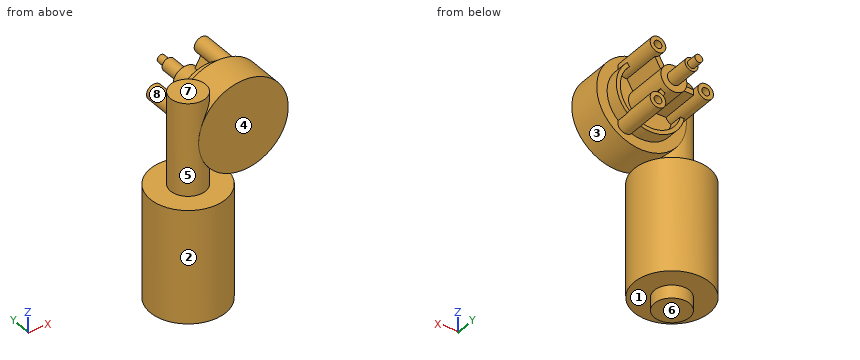
```python
from build123d import *

# Parameters (mm, degrees)
SKETCH1_R           = 29
BOSS_EXTRUDE1_DEPTH = 87
SKETCH3_W           = 13.5
SKETCH3_H           = 168
SKETCH4_R           = 34.5
BOSS_EXTRUDE2_DEPTH = 13.5
SKETCH5_R           = 6
SKETCH5_R_2         = 10
BOSS_EXTRUDE3_DEPTH = 35
BOSS_EXTRUDE4_DEPTH = 30
SKETCH7_R           = 26.5
SKETCH7_R_2         = 23.5
BOSS_EXTRUDE5_DEPTH = 10
SKETCH8_R           = 3
CUT_EXTRUDE1_DEPTH  = 18
SKETCH9_R           = 5
BOSS_EXTRUDE6_DEPTH = 19
SKETCH10_R          = 3
BOSS_EXTRUDE7_DEPTH = 8


with BuildPart() as part:
    # Sketch1 → Boss-Extrude1 (new body)
    with BuildSketch(Plane.XY):
        Circle(SKETCH1_R)
    extrude(amount=BOSS_EXTRUDE1_DEPTH)

    # Sketch3 → Revolve1 (revolve)
    with BuildSketch(Plane(origin=(0, 0, 0), x_dir=(1, 0, 0), z_dir=(0, 1, 0))):
        with Locations((-6.75, -74)):
            Rectangle(SKETCH3_W, SKETCH3_H)
    revolve(axis=Axis((0, 0, 0), (0, 0, 1)))

    # Sketch4 → Boss-Extrude2 (add, symmetric)
    with BuildSketch(Plane(origin=(0, 0, 0), x_dir=(1, 0, 0), z_dir=(0, 1, 0))):
        with Locations((33, -126.5)):
            Circle(SKETCH4_R)
    extrude(amount=BOSS_EXTRUDE2_DEPTH, both=True)

    # Sketch5 → Boss-Extrude3 (add)
    with BuildSketch(Plane(origin=(0, 13.5, 0), x_dir=(1, 0, 0), z_dir=(0, 1, 0))):
        with Locations((8.5, -126.5)):
            Circle(SKETCH5_R)
        with Locations((33, -126.5)):
            Circle(SKETCH5_R_2)
        with Locations((45.25, -105.282377607)):
            Circle(SKETCH5_R)
        with Locations((45.25, -147.717622393)):
            Circle(SKETCH5_R)
    extrude(amount=BOSS_EXTRUDE3_DEPTH)

    # Sketch6 → Boss-Extrude4 (add)
    with BuildSketch(Plane(origin=(0, 13.5, 0), x_dir=(1, 0, 0), z_dir=(0, 1, 0))):
        Polygon((31.845299462, -128.5), (2.843145751, -128.5), (2.843145751, -124.5), (31.845299462, -124.5), (46.346376317, -99.383398122), (49.810477932, -101.383398122), (36.0121545, -125.282795366), (36.116305102, -127.897598768), (49.810477932, -151.616601878), (46.346376317, -153.616601878), align=None)
    extrude(amount=BOSS_EXTRUDE4_DEPTH)

    # Sketch7 → Boss-Extrude5 (add)
    with BuildSketch(Plane(origin=(0, 13.5, 0), x_dir=(1, 0, 0), z_dir=(0, 1, 0))):
        with Locations((33, -126.5)):
            Circle(SKETCH7_R)
        with Locations((33, -126.5)):
            Circle(SKETCH7_R_2, mode=Mode.SUBTRACT)
    extrude(amount=BOSS_EXTRUDE5_DEPTH)

    # Sketch8 → Cut-Extrude1 (cut)
    with BuildSketch(Plane(origin=(0, 48.5, 0), x_dir=(1, 0, 0), z_dir=(0, 1, 0))):
        with Locations((8.5, -126.5)):
            Circle(SKETCH8_R)
        with Locations((45.25, -105.282377607)):
            Circle(SKETCH8_R)
        with Locations((45.25, -147.717622393)):
            Circle(SKETCH8_R)
    extrude(amount=-CUT_EXTRUDE1_DEPTH, mode=Mode.SUBTRACT)

    # Sketch9 → Boss-Extrude6 (add)
    with BuildSketch(Plane(origin=(0, 48.5, 0), x_dir=(1, 0, 0), z_dir=(0, 1, 0))):
        with Locations((33, -126.5)):
            Circle(SKETCH9_R)
    extrude(amount=BOSS_EXTRUDE6_DEPTH)

    # Sketch10 → Boss-Extrude7 (add)
    with BuildSketch(Plane(origin=(0, 67.5, 0), x_dir=(1, 0, 0), z_dir=(0, 1, 0))):
        with Locations((33, -126.5)):
            Circle(SKETCH10_R)
    extrude(amount=BOSS_EXTRUDE7_DEPTH)


solid = part.part
```
Input: part model. Units: mm. Frame: model coordinates. Face numbers are marked on the shaded views. A direction names the side the tool comes from. Coordinates: 2 decimals unless noted, no trailing zeros. Write each loop counter-clockwise with the first axis right and the second up, starting at its lowest first coordinate (ties: lowest second). Pieces come first, ordered by that corner, then holes.
1) Pin query (flat end, axial travel): pin 1 Ø5 at (x, z) = (-13.5, 31.5) entering from +Y; pin 2 Ø6.5 at (x, z) = (44, 106) entering from +Y; pin 3 Ø5 at (x, z) = (54.5, 134.5) entering from +Y. Return the tip coordinate at first contact, or that it passes through.
2) Section C-C on y = -5.5. Output: boundary loops of the cut face in (x, z), and give its area (3 significant figures).
3) Material intervals for line 1 along X through (y, z) = (44, 126); line 2 along Z through (x, y) = (45.25, 37); line 3 along X through (y, z) = (42.5, 126.5), sorted ascending.
4) Set-up query: the marked faces 4, 5, 6, 7 and 8. Return all of +Z, -Z, +X, -X, +Y, -Y with unobstructed straight access to the full face (end or side cutting, diameter ignored); none if empty.
5) Section D-D on z = 2. Output: boundary loops of the cut face in (x, y).
6) Section B-B on y = 18.5. Output: boundary loops of the cut face in (x, z), and give its area (3 significant figures).
7) Mould query, pull axis X, two halves, no side actions, for the marked faces 1, 2 and 3. Classes: pulls with the +X half, pulls with the -X half, needs draft (parallel to the pull), parting line crosses it, or undercut.
Check result:
1. pin 1: stops at y = 26.83
1. pin 2: stops at y = 48.5
1. pin 3: stops at y = 23.5
2. outline: (-28.47, 0) - (-12.33, 0) - (-12.33, -10) - (12.33, -10) - (12.33, 0) - (28.47, 0) - (28.47, 87) - (12.33, 87) - (12.33, 98.88) arc R34.5 ccw (long way) to (12.33, 154.12) - (12.33, 158) - (-12.33, 158) - (-12.33, 87) - (-28.47, 87) - close
2. area: 10,200 mm2
3. line 1: x = 2.52 to 5.54, 11.46 to 14.48, 23.01 to 42.99
3. line 2: z = 99.28 to 102.28, 108.28 to 111.28, 141.72 to 144.72, 150.72 to 153.72
3. line 3: x = 2.5 to 5.5, 11.5 to 43
4. face 4: +Z, +X, -X, -Y
4. face 5: none
4. face 6: -Z, +X, -X, +Y, -Y
4. face 7: +Z, -X, +Y, -Y
4. face 8: +Y
5. outline: circle Ø58 at (0, 0)
6. outline: (-22.33, 0) - (22.33, 0) - (22.33, 87) - (-22.33, 87) - close; (7.15, 120.65) arc R26.5 ccw to (40.86, 101.19) arc R6 ccw to (50.99, 107.04) arc R26.5 ccw to (50.99, 145.96) arc R6 ccw to (40.86, 151.81) arc R26.5 ccw to (7.15, 132.35) arc R6 ccw to start; hole (10.21, 120.75) arc R23.5 ccw to (39.41, 103.89) arc R6 cw to (40.69, 109.18) - (36.17, 117.01) arc R10 cw to (23.2, 124.5) - (14.16, 124.5) arc R6 cw to start; hole (10.21, 132.25) arc R6 cw to (14.16, 128.5) - (23.2, 128.5) arc R10 cw to (36.17, 135.99) - (40.69, 143.82) arc R6 cw to (39.41, 149.11) arc R23.5 ccw to start; hole (39.63, 119.01) - (44.15, 111.18) arc R6 cw to (49.37, 109.64) arc R23.5 ccw to (49.37, 143.36) arc R6 cw to (44.15, 141.82) - (39.63, 133.99) arc R10 cw to start
6. area: 5,010 mm2
7. face 1: needs draft
7. face 2: parting line crosses it
7. face 3: undercut
